Verification items for the finished model (mm, model axes). A direction names the side the tool comes from. Give positions to 0.01 mm unless a question says otherwise; leave off trailing zeros. Write each loop counter-clockwise with the first axis right and the second up, starting at its lowest first coordinate (ties: lowest second). Pieces come first, ordered by that corner, then holes. Notation, with made-up numbers: M 74.5,80.5 L 101.5,80.5 A23 ccw 101.5,97.5 Z; hole C 89,2.25 d3. An arc over 180 degrees is marked long. Write item = value, one per line.
from build123d import *

# Parameters (mm, degrees)
F0_W          = 101.6
F0_H          = 30.48
F1_DEPTH      = 10.16
F1_DEPTH_BACK = 10.16
F3_DEPTH      = 25.4
F4_R          = 5.08
F5_R          = 2.54


with BuildPart() as f1:
    # F0 (on Top) → F1 (new body, two sides)
    with BuildSketch(Plane.XY) as f1_sk:
        Rectangle(F0_W, F0_H)
    extrude(amount=F1_DEPTH)
    extrude(f1_sk.sketch, amount=-F1_DEPTH_BACK)

    # F2 (on face) → F3 (cut)
    with BuildSketch(Plane.XY.offset(10.16)):
        Polygon((37.4322741568, -15.24), (24.0645483136, -11.43), (-50.8, -11.43), (-50.8, -15.24), align=None)
        Polygon((35.8814075589, 15.24), (50.8, 0), (50.8, 15.24), align=None)
        Polygon((-50.8, 15.24), (-50.8, 11.43), (24.0645483136, 11.43), (35.8814075589, 15.24), align=None)
        Polygon((-50.8, -15.24), (-50.8, -11.43), (-50.8, 11.43), (-50.8, 15.24), (35.8814075589, 15.24), (50.8, 15.24), (50.8, 0), (61.7307946086, 0), (61.7307946086, 22.9567158967), (-64.5619183779, 22.9567158967), (-64.5619183779, -22.5874371827), (63.700273633, -22.5874371827), (50.8, -15.24), (37.4322741568, -15.24), align=None)
    extrude(amount=-F3_DEPTH, mode=Mode.SUBTRACT)

    # F4
    f4_edges = [f1.edges().sort_by_distance(p)[0] for p in [
        (35.881408, 15.24, 0),
        (24.064548, 11.43, 0),
        (50.8, -15.24, 0),
        (37.432274, -15.24, 0),
        (24.064548, -11.43, 0),
        (-50.8, -11.43, 0),
        (-50.8, 11.43, 0),
        (50.8, 0, 0),
    ]]
    fillet(f4_edges, radius=F4_R)

    # F5
    f5_edges = [f1.edges().sort_by_distance(p)[0] for p in [
        (30.748411, -13.335, -10.16),
        (37.439103, -15.191126, -10.16),
        (24.057719, -11.478874, -10.16),
        (41.931039, -15.24, -10.16),
        (-11.182628, -11.43, -10.16),
        (49.312102, -13.752102, -10.16),
        (-49.312102, -9.942102, -10.16),
        (50.8, -6.116281, -10.16),
        (-50.8, 0, -10.16),
        (50.4236, -0.153565, -10.16),
        (-49.312102, 9.942102, -10.16),
        (43.714908, 7.237734, -10.16),
        (-11.227078, 11.43, -10.16),
        (35.667245, 14.372668, -10.16),
        (24.054856, 11.491648, -10.16),
        (28.857652, 12.975396, -10.16),
        (30.748411, -13.335, 10.16),
        (37.439103, -15.191126, 10.16),
        (24.057719, -11.478874, 10.16),
        (41.931039, -15.24, 10.16),
        (-11.182628, -11.43, 10.16),
        (49.312102, -13.752102, 10.16),
        (-49.312102, -9.942102, 10.16),
        (50.8, -6.116281, 10.16),
        (-50.8, 0, 10.16),
        (50.4236, -0.153565, 10.16),
        (-49.312102, 9.942102, 10.16),
        (43.714908, 7.237734, 10.16),
        (-11.227078, 11.43, 10.16),
        (35.667245, 14.372668, 10.16),
        (24.054856, 11.491648, 10.16),
        (28.857652, 12.975396, 10.16),
    ]]
    fillet(f5_edges, radius=F5_R)


solid = f1.part
1) Tool access check on faces 1 (the flat face through (-12, 11.43, 0)), 2 (the cylindrical face through (-11.7, -10.7, -9.4)), 3 (the cylindrical face through (-10.7, 10.7, -9.4)), 4 (the flat face through (-11, -11.43, 0)). Record the directions out of +Z, -Z, +X, -X, +Y, -Y that give a thin tool (end or side, any length) a straight path to the whole face; none if there is none.
From the geometry:
face_1 = +Z, -Z, -X, +Y
face_2 = -Z, -X, -Y
face_3 = -Z, -X, +Y
face_4 = +Z, -Z, -X, -Y
2) Cross-section at B-B on z = 4.75. Record the boundary of the cut face in (x, y).
From the geometry:
outline = M -50.8,-6.35 A5.08 ccw -45.72,-11.43 L 23.35,-11.43 A5.08 cw 24.75,-11.62 L 36.75,-15.05 A5.08 ccw 38.14,-15.24 L 45.72,-15.24 A5.08 ccw 50.8,-10.16 L 50.8,-2.07 A5.08 ccw 49.35,1.48 L 38.08,12.99 A5.08 ccw 32.89,14.28 L 24.82,11.68 A5.08 cw 23.27,11.43 L -45.72,11.43 A5.08 ccw -50.8,6.35 Z
3) Depth check by flat-ended pin: P1, Ø10, axis at x = 29.5, z = 6.5, coming from the -Y side; P2, Ø4, axis at x = -6.5, z = -2.5, coming from the -Y side; P3, Ø8, axis at y = 4, z = 2, coming from the +X side; P4, Ø10, axis at x = -20.5, y = 10, coming from the -Z side. Enter the tip coordinate at first touch or a pass-through.
From the geometry:
P1 = -14.4
P2 = -11.43
P3 = 50.36
P4 = -10.16
4) Material ranges on probe 1 along Y at (x, z) = (-42, -0.75); probe 2 along X at (y, z) = (-5.25, 7.75); probe 3 along X at (y, z) = (3, 6.5), recorded low to high. Write a range as from..to.
From the geometry:
probe_1 = -11.43..11.43
probe_2 = -50.8..50.8
probe_3 = -50.8..47.86
5) Cross-section at A-A on x = -2.5. Record the boundary of the cut face in (y, z).
From the geometry:
outline = M -11.43,-7.62 A2.54 ccw -8.89,-10.16 L 8.89,-10.16 A2.54 ccw 11.43,-7.62 L 11.43,7.62 A2.54 ccw 8.89,10.16 L -8.89,10.16 A2.54 ccw -11.43,7.62 Z
